```python
from build123d import *

# Parameters (mm, degrees)
F0_W     = 75
F0_H     = 2
F0_W_2   = 80
F0_H_2   = 10
F1_DEPTH = 1.59
F2_R     = 2
F3_R     = 0.99999


# Not quite as in the source:
# - a fillet or chamfer is up to 0.001 mm smaller than in the source, because OpenCascade refuses the exact size


with BuildPart() as f1:
    # F0 (on Top) → F1 (new body)
    with BuildSketch(Plane.XY):
        Polygon((45, 0), (-45, 0), (-60, 0), (-60, -30), (-45, -30), (-45, -45), (45, -45), (45, -30), (60, -30), (60, 0), align=None)
        with Locations((0, -38.175)):
            Rectangle(F0_W, F0_H, mode=Mode.SUBTRACT)
        with Locations((0, -17.5)):
            Rectangle(F0_W_2, F0_H_2, mode=Mode.SUBTRACT)
    extrude(amount=F1_DEPTH)

    # F2
    f2_edges = [f1.edges().sort_by_distance(p)[0] for p in [
        (40, -22.5, 0.795),
        (-40, -12.5, 0.795),
        (40, -12.5, 0.795),
        (-40, -22.5, 0.795),
    ]]
    fillet(f2_edges, radius=F2_R)

    # F3 (radius 1 in the source; OpenCascade refuses exactly that, so slightly less here)
    f3_edges = [f1.edges().sort_by_distance(p)[0] for p in [
        (-37.5, -37.175, 0.795),
        (37.5, -37.175, 0.795),
        (37.5, -39.175, 0.795),
        (-37.5, -39.175, 0.795),
    ]]
    fillet(f3_edges, radius=F3_R)


solid = f1.part
```
The model under review builds one solid part; all positions refer to its coordinate system, in mm. A direction names the side the tool comes from. Coordinates: 2 decimals unless noted, no trailing zeros. Write each loop counter-clockwise with the first axis right and the second up, starting at its lowest first coordinate (ties: lowest second). Pieces come first, ordered by that corner, then holes. Notation, with made-up numbers: (-9.5, 14) -> (8.5, 14) arc R5 ccw to (8.5, 20) -> close; hole circle Ø2 at (-33, 59). An arc over 180 degrees is marked (long way). One line per item, written item: value. Start each with the question number.
Q1. For faces 1 (the face through (-1, -27, 1.59)), 2 (the face through (39.4, -21.93, 0.81)), list the 3-axis set-ups (+Z, -Z, +X, -X, +Y, -Y) from which the entire face can be reached by the end or side of a thin tool; tool diameter is ignored.
Q2. Add section A-A, the plane z = 1.1. Count the separate pieces of the cut face and the enclosed holes in it, then the cut area to 3 significant figures.
Q3. Add section C-C, the plane y = -41. Give the boundary of the cut face in (x, z), then the cut area to 3 significant figures.
Q4. Clearance check with flat-ended pins moving along their axes: P1, Ø0.5, axis at x = 50.5, z = 1, coming from the -Y side; P2, Ø1.5, axis at x = -1.5, y = -38, coming from the -Z side. State where each tip first meets the part, or that it passes through.
Q5. Add section D-D, the plane x = 51.5. Give the boundary of the cut face in (y, z), then the cut area to 3 significant figures.
Q6. To check wall thickness, follow probe 1 along Y at (x, z) = (-17, 1.2) (3 decimals); probe 2 along X at (y, z) = (-38, 0.5); probe 3 along X at (y, z) = (-39.5, 0.75). State the ranges of each line that lie inside material, in increasing order.
Q7. Add section B-B, the plane x = -19. Give the boundary of the cut face in (y, z) (3 decimals), then the cut area to 3 significant figures.
Q8. The part is to be moulded in two halves that separate along X. For faces 3 (the face through (-1, -27, 0)), 4 (the face through (-39.4, -21.93, 0.81)), say which applies: +X half, -X half, draft (parallel to the pull), parting line (faces both ways), or undercut.
Response:
1. face 1: +Z, +X, -X, +Y, -Y
1. face 2: +Z, -Z
2. separate pieces: 1
2. enclosed holes: 2
2. area: 4,000 mm²
3. outline: (-45, 0) -> (45, 0) -> (45, 1.59) -> (-45, 1.59) -> close
3. area: 143 mm²
4. P1: y = -30
4. P2: through
5. outline: (-30, 0) -> (0, 0) -> (0, 1.59) -> (-30, 1.59) -> close
5. area: 47.7 mm²
6. probe 1: -45 to -39.175, -37.175 to -22.5, -12.5 to 0
6. probe 2: -45 to -37.48, 37.48 to 45
6. probe 3: -45 to 45
7. outline: (-45, 0) -> (-39.175, 0) -> (-39.175, 1.59) -> (-45, 1.59) -> close; (-37.175, 0) -> (-22.5, 0) -> (-22.5, 1.59) -> (-37.175, 1.59) -> close; (-12.5, 0) -> (0, 0) -> (0, 1.59) -> (-12.5, 1.59) -> close
7. area: 52.5 mm²
8. face 3: draft
8. face 4: undercut
